For this review, take the finished solid that the model builds, in its own axes (mm). A direction names the side the tool comes from. Give positions to 0.01 mm unless a question says otherwise; leave off trailing zeros. Loops run counter-clockwise (first coordinate to the right, second up) from the corner with the lowest first, then second, coordinate; pieces in that order, holes last. Notation, with made-up numbers: (89.25, -6) -> (103.25, -6) arc R37 ccw to (103.25, 30) -> close; hole circle Ø4 at (-20, 62). An arc over 180 degrees is marked (long way). Write each question's results on one line, items separated by ' | '. Start each with the question number.
```python
from build123d import *

# Parameters (mm, degrees)
SKETCH1_W           = 60
SKETCH1_H           = 4
BOSS_EXTRUDE1_DEPTH = 45
SKETCH1_3_R         = 2.2
BOSS_EXTRUDE2_DEPTH = 5
SKETCH2_R           = 3
SKETCH2_R_2         = 1.6
CUT_EXTRUDE1_DEPTH  = 5
BOSS_EXTRUDE3_DEPTH = 45
FILLET1_R           = 2.5
FILLET3_R           = 2.5
SKETCH3_R           = 4
BOSS_EXTRUDE4_DEPTH = 12
SKETCH4_R           = 6
BOSS_EXTRUDE5_DEPTH = 5
FILLET4_R           = 1


with BuildPart() as part:
    # Sketch1 → Boss-Extrude1 (new body)
    with BuildSketch(Plane.XY):
        with Locations((-82.025641026, 5.685176195)):
            Rectangle(SKETCH1_W, SKETCH1_H)
    extrude(amount=BOSS_EXTRUDE1_DEPTH)

    # Sketch1_3 → Boss-Extrude2 (add)
    with BuildSketch(Plane.XY):
        Polygon((-112.025641026, 27.185176195), (-112.025641026, 7.685176195), (-103.025641026, 7.685176195), (-103.025641026, 27.185176195), (-103.025641026, 31.685176195), (-112.025641026, 31.685176195), align=None)
        with Locations((-106.025641026, 14.685176195)):
            Circle(SKETCH1_3_R, mode=Mode.SUBTRACT)
        with Locations((-106.025641026, 24.685176195)):
            Circle(SKETCH1_3_R, mode=Mode.SUBTRACT)
        Polygon((-61.025641026, 27.185176195), (-61.025641026, 7.685176195), (-52.025641026, 7.685176195), (-52.025641026, 27.185176195), (-52.025641026, 31.685176195), (-61.025641026, 31.685176195), align=None)
        with Locations((-58.025641026, 14.685176195)):
            Circle(SKETCH1_3_R, mode=Mode.SUBTRACT)
        with Locations((-58.025641026, 24.685176195)):
            Circle(SKETCH1_3_R, mode=Mode.SUBTRACT)
    extrude(amount=BOSS_EXTRUDE2_DEPTH)

    # Sketch2 → Cut-Extrude1 (cut, through all)
    with BuildSketch(Plane(origin=(0, 7.685176195, 0), x_dir=(1, 0, 0), z_dir=(0, 1, 0))):
        with Locations((-82.025641026, -31)):
            Circle(SKETCH2_R)
        with Locations((-77.025641026, -26)):
            Circle(SKETCH2_R_2)
        with Locations((-87.025641026, -26)):
            Circle(SKETCH2_R_2)
        with Locations((-77.025641026, -36)):
            Circle(SKETCH2_R_2)
        with Locations((-87.025641026, -36)):
            Circle(SKETCH2_R_2)
    extrude(amount=-CUT_EXTRUDE1_DEPTH, mode=Mode.SUBTRACT)

    # Sketch1_4 → Boss-Extrude3 (add)
    with BuildSketch(Plane.XY):
        Polygon((-112.025641026, 35.685176195), (-112.025641026, 31.685176195), (-103.025641026, 31.685176195), (-61.025641026, 31.685176195), (-52.025641026, 31.685176195), (-52.025641026, 35.685176195), align=None)
    extrude(amount=BOSS_EXTRUDE3_DEPTH)

    # Fillet1
    fillet1_edges = [part.edges().sort_by_distance(p)[0] for p in [
        (-112.025641026, 5.685176195, 45),
        (-52.025641026, 5.685176195, 45),
        (-112.025641026, 33.685176195, 45),
        (-52.025641026, 33.685176195, 45),
    ]]
    fillet(fillet1_edges, radius=FILLET1_R)

    # Fillet3
    fillet3_edges = [part.edges().sort_by_distance(p)[0] for p in [
        (-107.525641026, 31.685176195, 5),
        (-107.525641026, 7.685176195, 5),
        (-56.525641026, 31.685176195, 5),
        (-56.525641026, 7.685176195, 5),
    ]]
    fillet(fillet3_edges, radius=FILLET3_R)

    # Sketch3 → Boss-Extrude4 (add)
    with BuildSketch(Plane(origin=(0, 35.685176195, 0), x_dir=(1, 0, 0), z_dir=(0, 1, 0))):
        with Locations((-82.025641026, -31)):
            Circle(SKETCH3_R)
    extrude(amount=BOSS_EXTRUDE4_DEPTH)

    # Sketch4 → Boss-Extrude5 (add)
    with BuildSketch(Plane(origin=(0, 35.685176195, 0), x_dir=(1, 0, 0), z_dir=(0, 1, 0))):
        with Locations((-82.025641026, -31)):
            Circle(SKETCH4_R)
    extrude(amount=BOSS_EXTRUDE5_DEPTH)

    # Fillet4
    fillet4_edges = [part.edges().sort_by_distance(p)[0] for p in [
        (-86.025641026, 40.685176195, 31),
    ]]
    fillet(fillet4_edges, radius=FILLET4_R)


solid = part.part
```
1. We need section D-D (y = 25.5). Write out the cut boundary in (x, z), plus the area to 3 significant figures.
2. For pin 1 Ø2.5 at (x, z) = (-87.03, 26) entering from -Y; pin 2 Ø8 at (y, z) = (23.5, 11.5) entering from +X; pin 3 Ø10 at (x, y) = (-58.5, 17) entering from +Z; pin 4 Ø3.5 at (x, z) = (-77.03, 26) entering from +Y, all flat-tipped, find the tip position at first contact; note any pin that passes through.
3. We need section C-C (x = -57). Write out the cut boundary in (y, z).
4. We need section B-B (z = 39). Write out the cut boundary in (x, y).
5. Draft analysis for pull direction Y (two halves, no side actions). For faces 1 (the flat face through (-108, 20, 5)), 2 (the flat face through (-86, 40.685, 27)), 3 (the flat face through (-82, 6, 45)), 4 (the flat face through (-82, 31.685, 22)), state which applies: released by +Y, released by -Y, zero draft, split by the parting line, or undercut.
6. Machinability: for faces 5 (the cylindrical face through (-75.5, 5.71, 25.52)), 6 (the cylindrical face through (-111.31, 33.66, 44.25)), 7 (the cylindrical face through (-107.59, 30.97, 5.75)), 8 (the cylindrical face through (-86.79, 38.15, 34.65)), 9 (the flat face through (-61.026, 20, 3)), which of the approach directions +Z, -Z, +X, -X, +Y, -Y give a long, thin tool a straight path to every point of the face, cutting with its end or side? Answer none if there is none.
7. Wall thickness on L1, parallel to X at y = 6, z = 36; L2, parallel to Y at x = -61, z = 37; L3, parallel to X at y = 4.9, z = 31: over which ranges is each line inside the solid? List them lowest first.
8. We need section A-A (x = -94). Write out the cut boundary in (y, z), plus the area to 3 significant figures.
Response:
1) outline: (-112.03, 0) -> (-108.07, 0) -> (-108.07, 5) -> (-112.03, 5) -> close; (-103.98, 0) -> (-103.03, 0) -> (-103.03, 5) -> (-103.98, 5) -> close; (-61.03, 0) -> (-60.07, 0) -> (-60.07, 5) -> (-61.03, 5) -> close; (-55.98, 0) -> (-52.03, 0) -> (-52.03, 5) -> (-55.98, 5) -> close | area: 49.1 mm2
2) pin 1: stops at y = 31.69 | pin 2: passes through | pin 3: stops at z = 5 | pin 4: stops at y = 40.69
3) outline: (3.69, 0) -> (12.74, 0) -> (12.74, 5) -> (10.19, 5) arc R2.5 cw to (7.69, 7.5) -> (7.69, 45) -> (3.69, 45) -> close; (16.63, 0) -> (22.74, 0) -> (22.74, 5) -> (16.63, 5) -> close; (26.63, 0) -> (35.69, 0) -> (35.69, 45) -> (31.69, 45) -> (31.69, 7.5) arc R2.5 cw to (29.19, 5) -> (26.63, 5) -> close
4) outline: (-112.03, 3.69) -> (-52.03, 3.69) -> (-52.03, 7.69) -> (-112.03, 7.69) -> close; (-112.03, 31.69) -> (-52.03, 31.69) -> (-52.03, 35.69) -> (-112.03, 35.69) -> close
5) face 1: undercut | face 2: released by +Y | face 3: zero draft | face 4: undercut
6) face 5: -Y | face 6: +Z, -X, +Y, -Y | face 7: +Z, +X, -X | face 8: +Y | face 9: +Z, -Z
7) L1: x = -112.03 to -88.63, -85.43 to -78.63, -75.43 to -52.03 | L2: y = 3.69 to 7.69, 31.69 to 35.69 | L3: x = -112.03 to -85.03, -79.03 to -52.03
8) outline: (3.69, 0) -> (7.69, 0) -> (7.69, 45) -> (3.69, 45) -> close; (31.69, 0) -> (35.69, 0) -> (35.69, 45) -> (31.69, 45) -> close | area: 360 mm2
